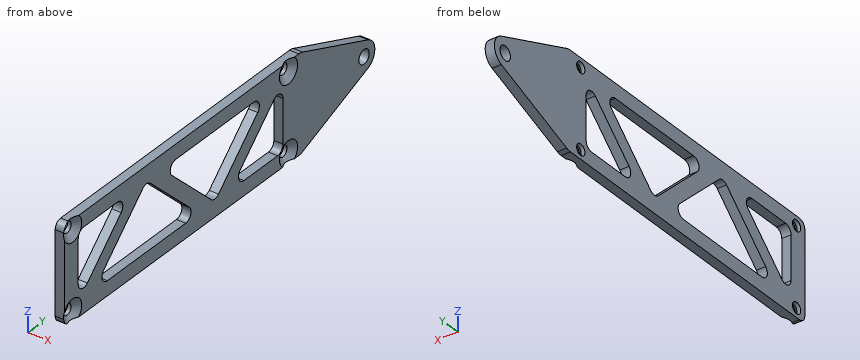
from build123d import *

# Parameters (mm, degrees)
SKETCH1_W                                 = 41.514809608
SKETCH1_H                                 = 98.81
SKETCH1_R                                 = 1.8288
SKETCH1_R_2                               = 2.413
BOSS_EXTRUDE1_DEPTH                       = 3.175
SKETCH2_W                                 = 4.112404804
SKETCH2_H                                 = 141.223
CUT_EXTRUDE1_DEPTH                        = 106.912542124
FILLET1_R                                 = 2.5
FILLET2_R                                 = 5
CSK_FOR_6_FLAT_HEAD_MACHINE_SCREW_2_COUNT = 2
CSK_FOR_6_FLAT_HEAD_MACHINE_SCREW_2_PITCH = 26.9494
CSK_FOR_6_FLAT_HEAD_MACHINE_SCREW_3_COUNT = 2
CSK_FOR_6_FLAT_HEAD_MACHINE_SCREW_3_PITCH = 103.567708096
CSK_FOR_6_FLAT_HEAD_MACHINE_SCREW_4_COUNT = 2
CSK_FOR_6_FLAT_HEAD_MACHINE_SCREW_4_PITCH = 100


with BuildPart() as part:
    # Sketch1 → Boss-Extrude1 (new body)
    # profile 1 of 6: a face of its own
    with BuildSketch(Plane(origin=(0, 0, 0), x_dir=(0, 0, -1), z_dir=(1, 0, 0))):
        with Locations((0, -54.405)):
            Rectangle(SKETCH1_W, SKETCH1_H)
        with Locations((13.4747, -100)):
            Circle(SKETCH1_R, mode=Mode.SUBTRACT)
        with Locations((-13.4747, -100)):
            Circle(SKETCH1_R, mode=Mode.SUBTRACT)
    # profile 2 of 6: a face of its own
    with BuildSketch(Plane(origin=(0, 0, 0), x_dir=(0, 0, -1), z_dir=(1, 0, 0))):
        Polygon((0, 48.916537522), (20.757404804, -5), (-20.757404804, -5), align=None)
        with Locations((13.4747, 0)):
            Circle(SKETCH1_R, mode=Mode.SUBTRACT)
        with Locations((0, 35)):
            Circle(SKETCH1_R_2, mode=Mode.SUBTRACT)
        with Locations((-13.4747, 0)):
            Circle(SKETCH1_R, mode=Mode.SUBTRACT)
    # profile 3 of 6: a face of its own
    with BuildSketch(Plane(origin=(0, 0, 0), x_dir=(0, 0, -1), z_dir=(1, 0, 0))):
        with Locations((-13.4747, 0)):
            Circle(SKETCH1_R)
    # profile 4 of 6: a face of its own
    with BuildSketch(Plane(origin=(0, 0, 0), x_dir=(0, 0, -1), z_dir=(1, 0, 0))):
        with Locations((13.4747, 0)):
            Circle(SKETCH1_R)
    # profile 5 of 6: a face of its own
    with BuildSketch(Plane(origin=(0, 0, 0), x_dir=(0, 0, -1), z_dir=(1, 0, 0))):
        with Locations((13.4747, -100)):
            Circle(SKETCH1_R)
    # profile 6 of 6: a face of its own
    with BuildSketch(Plane(origin=(0, 0, 0), x_dir=(0, 0, -1), z_dir=(1, 0, 0))):
        with Locations((-13.4747, -100)):
            Circle(SKETCH1_R)
    extrude(amount=BOSS_EXTRUDE1_DEPTH)

    # Sketch2 → Cut-Extrude1 (cut, through all)
    with BuildSketch(Plane(origin=(3.175, 0, 0), x_dir=(0, 0, -1), z_dir=(1, 0, 0))):
        Polygon((11.645, -2.5), (-11.645, -2.5), (11.645, -26.898674048), align=None)
        Polygon((-11.645, -9.741325952), (11.645, -34.14), (-11.645, -58.538674048), (-11.645, -34.14), align=None)
        Polygon((-11.645, -73.021325952), (-11.645, -97.42), (11.645, -97.42), align=None)
        Polygon((11.645, -41.381325952), (11.645, -65.78), (11.645, -90.178674048), (-11.645, -65.78), align=None)
        with Locations((-18.701202402, -33.1985)):
            Rectangle(SKETCH2_W, SKETCH2_H)
        with Locations((18.701202402, -33.1985)):
            Rectangle(SKETCH2_W, SKETCH2_H)
    extrude(amount=-CUT_EXTRUDE1_DEPTH, mode=Mode.SUBTRACT)

    # Fillet1
    fillet1_edges = [part.edges().sort_by_distance(p)[0] for p in [
        (1.5875, -103.81, -16.645),
        (1.5875, -9.741325952, 11.645),
        (1.5875, -34.14, -11.645),
        (1.5875, -58.538674048, 11.645),
        (1.5875, -26.898674048, -11.645),
        (1.5875, -2.5, 11.645),
        (1.5875, -2.5, -11.645),
        (1.5875, -90.178674048, -11.645),
        (1.5875, -65.78, 11.645),
        (1.5875, -41.381325952, -11.645),
        (1.5875, -103.81, 16.645),
        (1.5875, -73.021325952, 11.645),
        (1.5875, -97.42, -11.645),
        (1.5875, -97.42, 11.645),
    ]]
    fillet(fillet1_edges, radius=FILLET1_R)

    # Fillet2
    fillet2_edges = [part.edges().sort_by_distance(p)[0] for p in [
        (1.5875, 48.916537522, 0),
        (1.5875, 5.681808734, -16.645),
        (1.5875, 5.681808734, 16.645),
    ]]
    fillet(fillet2_edges, radius=FILLET2_R)

    # Sketch4 → CSK for #6 Flat Head Machine Screw (100)1 (revolve, cut)
    with BuildSketch(Plane(origin=(3.175, 0, 13.4747), x_dir=(0, 0, -1), z_dir=(0, 1, 0))):
        Polygon((0, 0), (0, 3.175), (1.89865, 3.175), (1.89865, 1.930031858), (4.1987724, 0), align=None)
    csk_for_6_flat_head_machine_screw_100 = revolve(axis=Axis((9.525, 0, 13.4747), (-1, 0, 0)), mode=Mode.SUBTRACT)

    # CSK for _6 Flat Head Machine Screw _ 2: CSK for #6 Flat Head Machine Screw (100)1 ×2
    with Locations(*[(0, 0, -i * CSK_FOR_6_FLAT_HEAD_MACHINE_SCREW_2_PITCH) for i in range(1, CSK_FOR_6_FLAT_HEAD_MACHINE_SCREW_2_COUNT)]):
        add(csk_for_6_flat_head_machine_screw_100, mode=Mode.SUBTRACT)

    # CSK for _6 Flat Head Machine Screw _ 3: CSK for #6 Flat Head Machine Screw (100)1 ×2
    with Locations(*[Vector(0, -0.9655519257685299, -0.2602104506830644) * (i * CSK_FOR_6_FLAT_HEAD_MACHINE_SCREW_3_PITCH) for i in range(1, CSK_FOR_6_FLAT_HEAD_MACHINE_SCREW_3_COUNT)]):
        add(csk_for_6_flat_head_machine_screw_100, mode=Mode.SUBTRACT)

    # CSK for _6 Flat Head Machine Screw _ 4: CSK for #6 Flat Head Machine Screw (100)1 ×2
    with Locations(*[(0, -i * CSK_FOR_6_FLAT_HEAD_MACHINE_SCREW_4_PITCH, 0) for i in range(1, CSK_FOR_6_FLAT_HEAD_MACHINE_SCREW_4_COUNT)]):
        add(csk_for_6_flat_head_machine_screw_100, mode=Mode.SUBTRACT)


solid = part.part
Geometry check sheet. Reference: the model listing, model coordinates, mm. Round coordinates to 2 decimals unless told otherwise and drop trailing zeros. Write each loop counter-clockwise with the first axis right and the second up, starting at its lowest first coordinate (ties: lowest second). Pieces come first, ordered by that corner, then holes.
Item 1: Section check B-B (z = 0). Record the boundary of the cut face in (x, y) (3 decimals), plus the area to 3 significant figures.
Determined:
outline: (0, -103.81) - (3.175, -103.81) - (3.175, -97.42) - (0, -97.42) - close; (0, -85.221) - (3.175, -85.221) - (3.175, -77.979) - (0, -77.979) - close; (0, -53.581) - (3.175, -53.581) - (3.175, -46.339) - (0, -46.339) - close; (0, -21.941) - (3.175, -21.941) - (3.175, -14.699) - (0, -14.699) - close; (0, -2.5) - (3.175, -2.5) - (3.175, 32.587) - (0, 32.587) - close; (0, 37.413) - (3.175, 37.413) - (3.175, 40) - (0, 40) - close
area: 209 mm2
Item 2: Go/stop test with flat-tipped pins: pin 1 Ø4.5 at (y, z) = (-100, -13.47) entering from +X; pin 2 Ø3 at (y, z) = (0, 13.47) entering from -X; pin 3 Ø1.6 at (x, z) = (1.5, 5) entering from +Y. Record where each tip stops, or that it passes through.
Determined:
pin 1: stops at x = 1.54
pin 2: passes through
pin 3: stops at y = 37.71
Item 3: Section check A-A (y = -91.5). Record the boundary of the cut face in (x, z) (3 decimals), plus the area to 3 significant figures.
Determined:
outline: (0, -16.645) - (3.175, -16.645) - (3.175, -5.994) - (0, -5.994) - close; (0, 11.645) - (3.175, 11.645) - (3.175, 16.645) - (0, 16.645) - close
area: 49.7 mm2
Item 4: Section check D-D (y = -74). Record the boundary of the cut face in (x, z) (3 decimals).
Determined:
outline: (0, -16.645) - (3.175, -16.645) - (3.175, -11.645) - (0, -11.645) - close; (0, 3.799) - (3.175, 3.799) - (3.175, 16.645) - (0, 16.645) - close
Item 5: Material ranges on line 1 along Z through (x, y) = (0.55, 0) (3 decimals); line 2 along Y through (x, z) = (1.25, -2.5); line 3 along Y through (x, z) = (2.3, -3), recorded low to high.
Determined:
line 1: z = -16.645 to -15.373, -11.576 to 11.576, 15.373 to 16.645
line 2: y = -103.81 to -97.42, -87.84 to -80.6, -50.96 to -43.72, -24.56 to -17.32, -2.5 to 39.33
line 3: y = -103.81 to -97.42, -88.36 to -81.12, -50.44 to -43.2, -25.08 to -17.84, -2.5 to 39
Item 6: Section check C-C (x = 0.5). Give the number of separate pieces and of enclosed holes in the cut face, plus the area to 3 significant figures.
Determined:
separate pieces: 1
enclosed holes: 9
area: 2,630 mm2
